Could you check a few things on this drawing? It's one solid part, dimensions in mm from its lowest x, y, z. A direction names the side the tool comes from. Coordinates: 2 decimals unless noted, no trailing zeros. Order: outer loops, then holes, each group sorted by start corner. A loop starts at its lowest first (then second) coordinate and runs counter-clockwise, first axis right, second up. Notation, with made-up numbers: (52, 50) -> (83, 50) arc R12 cw to (83, 68) -> close; hole circle Ø8 at (-2.75, 15.25). An arc over 180 degrees is marked (long way). Answer as CSV lines item,"result".
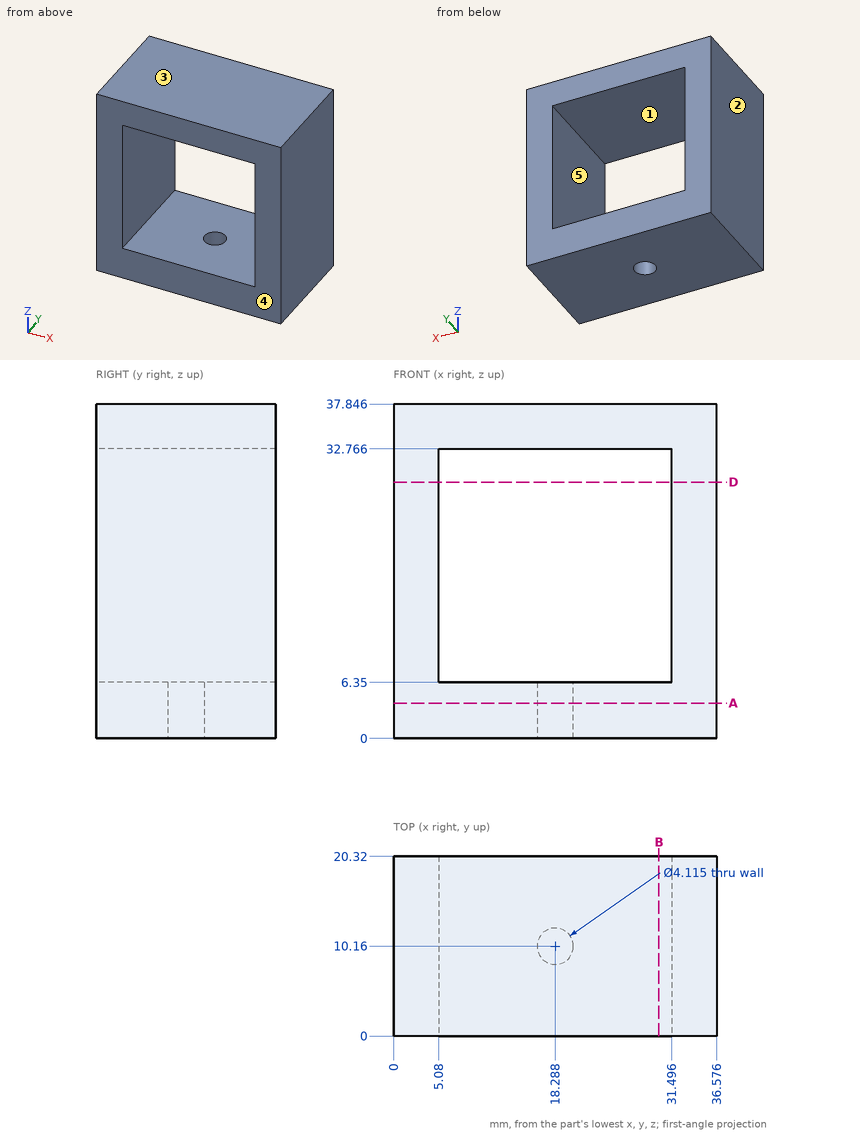
Q1. Imagine slicing it at A-A (z = 4). List the corners of the cut face in (x, y) for me (1 decimal), and give its area (3 significant figures).
Solution:
outline,"(0, 0) -> (36.6, 0) -> (36.6, 20.3) -> (0, 20.3) -> close; hole circle Ø4.1 at (18.3, 10.2)"
area,"730 mm2"
Q2. Imagine slicing it at B-B (x = 30). List the corners of the cut face in (y, z) for me.
Solution:
outline,"(0, 0) -> (20.32, 0) -> (20.32, 6.35) -> (0, 6.35) -> close; (0, 32.77) -> (20.32, 32.77) -> (20.32, 37.85) -> (0, 37.85) -> close"
Q3. Which directions (+Z, -Z, +X, -X, +Y, -Y) give clear straight access to the entire face, cutting with the end or side of a thin tool? Please do the marked faces 4 and 5.
Solution:
face 4,"+Z, -Z, +X, -X, -Y"
face 5,"+Y, -Y"
Q4. If I drill on line 1 (X direction, y = 2.25, z = 32); line 2 (Z direction, x = 29.5, y = 18.5), over which ranges is the centre line in solid material (lowest first)?
Solution:
line 1,"0 to 5.08, 31.5 to 36.58"
line 2,"0 to 6.35, 32.77 to 37.85"
Q5. Imagine slicing it at D-D (z = 29). List the corners of the cut face in (x, y) for me.
Solution:
outline,"(0, 0) -> (5.08, 0) -> (5.08, 20.32) -> (0, 20.32) -> close; (31.5, 0) -> (36.58, 0) -> (36.58, 20.32) -> (31.5, 20.32) -> close"
Q6. For P1, Ø12, axis at x = 21.5, z = 21.5, coming from the +Y side; P2, Ø10, axis at x = 15, y = 8, coming from the -Z side, each with a flat end and sliding along its axis, tell me the tip position at first contact or that it passes through.
Solution:
P1,"through"
P2,"z = 0"
Q7. We'd pull the mould along X, two halves only. Please class the marked faces 1, 2 and 3: pulls with the +X half, pulls with the -X half, needs draft (parallel to the pull), parting line crosses it, or undercut.
Solution:
face 1,"undercut"
face 2,"pulls with the -X half"
face 3,"needs draft"
